```python
from build123d import *

# Parameters (mm, degrees)
BOSS_EXTRUDE1_DEPTH = 25
SKETCH2_R           = 5
CUT_EXTRUDE1_DEPTH  = 25
SKETCH3_W           = 45.972937234
SKETCH3_H           = 12.458050792
CUT_EXTRUDE2_DEPTH  = 58.995783967
FILLET1_R           = 1


with BuildPart() as part:
    # Sketch1 → Boss-Extrude1 (new body)
    with BuildSketch(Plane(origin=(0, 0, 0), x_dir=(0, 0, -1), z_dir=(1, 0, 0))):
        Polygon((0, 0), (-45.972937234, 0), (-45.972937234, -15.228150532), (0, -25), align=None)
    extrude(amount=BOSS_EXTRUDE1_DEPTH)

    # Sketch2 → Cut-Extrude1 (cut)
    with BuildSketch(Plane(origin=(0, -23.919318221, 5.084208038), x_dir=(1, 0, 0), z_dir=(0, -0.9781476007338064, 0.20791169081775596))):
        with Locations(Location((12.5, 17.30220773, 0), (0, 0, 270))):
            Circle(SKETCH2_R)
    extrude(amount=-CUT_EXTRUDE1_DEPTH, mode=Mode.SUBTRACT)

    # Sketch3 → Cut-Extrude2 (cut, through all)
    with BuildSketch(Plane.ZY):
        with Locations((22.986468617, -6.229025396)):
            Rectangle(SKETCH3_W, SKETCH3_H)
    extrude(amount=-CUT_EXTRUDE2_DEPTH, mode=Mode.SUBTRACT)

    # Fillet1
    fillet1_edges = [part.edges().sort_by_distance(p)[0] for p in [
        (12.5, -12.458050792, 45.972937234),
        (12.5, -12.458050792, 0),
        (12.5, -25, 0),
        (12.5, -15.228150532, 45.972937234),
    ]]
    fillet(fillet1_edges, radius=FILLET1_R)


solid = part.part
```
Geometry: final body of the model. Coordinates: model frame, mm. Round coordinates to 2 decimals unless told otherwise and drop trailing zeros. Order: outer loops, then holes, each group sorted by start corner. A loop starts at its lowest first (then second) coordinate and runs counter-clockwise, first axis right, second up. Notation, with made-up numbers: (26.25, 0.25) -> (79.25, 0.25) arc R23 ccw to (79.25, 17.25) -> close; hole circle Ø2 at (-20, 36). An arc over 180 degrees is marked (long way). Use one line per item in the form item = value. Start each with the question number.
1. Line query: probe 1 along X at (y, z) = (-16, 18); probe 2 along Y at (x, z) = (4.75, 21); probe 3 along Z at (x, y) = (2.5, -14.5). Output: solid intervals per line, ascending.
2. Cut plane C-C (x = 8). Return the cut outline in (y, z).
3. Cut plane A-A (x = 3.75). Return the cut outline in (y, z).
4. Pin query (flat end, axial travel): pin 1 Ø1 at (x, z) = (14.5, 16) entering from -Y; pin 2 Ø1.5 at (x, z) = (4, 24) entering from -Y. Return the tip coordinate at first contact, or that it passes through.
5. Cut plane D-D (z = 3). Return the cut outline in (x, y).
6. Draft query along Z for faces 1 (the face through (14, -16.92, 16.41)), 2 (the face through (12, -14, 45.973)), 3 (the face through (25, -17, 18)). Return one class per face: pulls with the +Z half, pulls with the -Z half, needs draft (parallel to the pull), parting line crosses it, or undercut.
7. Cut plane B-B (x = 15.75). Return the cut outline in (y, z).
Solution:
q1.probe_1 = 0 to 8.52, 16.48 to 25
q1.probe_2 = -20.54 to -12.46
q1.probe_3 = 0 to 45.97
q2.outline = (-24.74, 1.21) arc R1 ccw to (-23.77, 0) -> (-13.46, 0) arc R1 ccw to (-12.46, 1) -> (-12.46, 18.11) -> (-20.78, 19.88) -> close; (-19.87, 24.14) -> (-12.46, 22.56) -> (-12.46, 44.97) arc R1 ccw to (-13.46, 45.97) -> (-14.42, 45.97) arc R1 ccw to (-15.4, 45.18) -> close
q3.outline = (-24.74, 1.21) arc R1 ccw to (-23.77, 0) -> (-13.46, 0) arc R1 ccw to (-12.46, 1) -> (-12.46, 44.97) arc R1 ccw to (-13.46, 45.97) -> (-14.42, 45.97) arc R1 ccw to (-15.4, 45.18) -> close
q4.pin_1 = -21.71
q4.pin_2 = -20.06
q5.outline = (0, -24.36) -> (25, -24.36) -> (25, -12.46) -> (0, -12.46) -> close
q6.face_1 = undercut
q6.face_2 = pulls with the +Z half
q6.face_3 = needs draft
q7.outline = (-24.74, 1.21) arc R1 ccw to (-23.77, 0) -> (-13.46, 0) arc R1 ccw to (-12.46, 1) -> (-12.46, 16.45) -> (-21.11, 18.29) -> close; (-19.53, 25.72) -> (-12.46, 24.22) -> (-12.46, 44.97) arc R1 ccw to (-13.46, 45.97) -> (-14.42, 45.97) arc R1 ccw to (-15.4, 45.18) -> close
